from build123d import *

# Parameters (mm, degrees)
F1_R   = 213
F1_R_2 = 203


with BuildPart() as f2:
    # F2: sweep along a path in F0
    with BuildLine(Plane.XZ) as f2_path:
        Line((0, 0), (0, -183.805903785))
        Line((0, -183.805903785), (139.1482145694, -519.7394105784))
        Line((139.1482145694, -519.7394105784), (396.2605894216, -776.8517854306))
        Line((396.2605894216, -776.8517854306), (732.194096215, -916))
        Line((732.194096215, -916), (1100, -916))
    # F1 (on Top) → F2 (sweep)
    with BuildSketch(Plane.XY):
        Circle(F1_R)
        Circle(F1_R_2, mode=Mode.SUBTRACT)
    sweep(path=f2_path.line, transition=Transition.RIGHT)


solid = f2.part
The model under review builds one solid part; all positions refer to its coordinate system, in mm. A direction names the side the tool comes from. Give positions to 0.01 mm unless a question says otherwise; leave off trailing zeros. Loops run counter-clockwise (first coordinate to the right, second up) from the corner with the lowest first, then second, coordinate; pieces in that order, holes last. Notation, with made-up numbers: (38, 83.5) -> (48, 83.5) arc R16 cw to (48, 87.5) -> close; hole circle Ø8 at (75, 72). An arc over 180 degrees is marked (long way). Put each result on its own line as item: value. Start each with the question number.
1. We need section A-A on y = 0. State the section outline as (x, z) points, then the cut area to 3 significant figures.
2. We need section B-B on x = 842. State the section outline as (y, z) points, then the cut area to 3 significant figures.
3. We need section C-C on y = -134.5. State the section outline as (x, z) points, then the cut area to 3 significant figures.
4. Wall thickness on probe 1 along Y at (x, z) = (0, -99); probe 2 along Z at (x, y) = (214, -129.5); probe 3 along X at (y, z) = (2.5, -506): over which ranges is each line inside the solid? List them lowest first.
5. Clearance check with flat-ended pins moving along their axes: P1, Ø4, axis at y = 24, z = -774.5, coming from the +X side; P2, Ø4, axis at y = -105.5, z = -609, coming from the +X side; P3, Ø5, axis at y = -158, z = -221.5, coming from the +X side. State where each tip first meets the part, or that it passes through.
6. Mouldability with a two-part tool opening along Z and no side actions: class faces 1 (the face through (1100, 78, -1104)), 2 (the face through (897.784, -9.365, -1128.794)), 3 (the face through (-116.6, -8.93, -432.26)), 4 (the face through (489.49, -8.93, -1034.98)) as released by +Z, released by -Z, zero draft, split by the parting line, or undercut.
7. For faces 5 (the face through (-212.794, -9.365, -89.54)), 6 (the face through (898.765, -8.926, -1118.804)), 7 (the face through (-125.821, -9.365, -436.105)), list the 3-axis set-ups (+Z, -Z, +X, -X, +Y, -Y) from which the entire face can be reached by the end or side of a thin tool; tool diameter is ignored.
Determined:
1. outline: (-213, -226.17) -> (-41.42, -640.39) -> (275.61, -957.42) -> (689.83, -1129) -> (1100, -1129) -> (1100, -1119) -> (691.81, -1119) -> (281.27, -948.95) -> (-32.95, -634.73) -> (-203, -224.19) -> (-203, 0) -> (-213, 0) -> close; (203, -143.43) -> (311.24, -404.75) -> (511.25, -604.76) -> (772.57, -713) -> (1100, -713) -> (1100, -703) -> (774.56, -703) -> (516.92, -596.28) -> (319.72, -399.08) -> (213, -141.44) -> (213, 0) -> (203, 0) -> close
1. area: 32,800 mm^2
2. outline: circle Ø426 at (0, -916); hole circle Ø406 at (0, -916)
2. area: 13,100 mm^2
3. outline: (-165.16, -216.66) -> (-0.87, -613.3) -> (302.7, -916.87) -> (699.34, -1081.16) -> (1100, -1081.16) -> (1100, -1068.05) -> (701.95, -1068.05) -> (310.13, -905.75) -> (10.25, -605.87) -> (-152.05, -214.05) -> (-152.05, 0) -> (-165.16, 0) -> close; (152.05, -153.56) -> (268.05, -433.61) -> (482.39, -647.95) -> (762.44, -763.95) -> (1100, -763.95) -> (1100, -750.84) -> (765.05, -750.84) -> (489.82, -636.83) -> (279.17, -426.18) -> (165.16, -150.95) -> (165.16, 0) -> (152.05, 0) -> close
3. area: 43,100 mm^2
4. probe 1: -213 to -203, 203 to 213
4. probe 2: -833.75 to -815.67, -291.94 to -258.54
4. probe 3: -97.08 to -86.25, 412.47 to 426.62
5. P1: x = 110.87
5. P2: x = 492.65
5. P3: x = 173.35
6. face 1: zero draft
6. face 2: split by the parting line
6. face 3: undercut
6. face 4: undercut
7. face 5: +Z
7. face 6: +X
7. face 7: none
